Build history of the part. All positions in model axes, mm. A direction names the side the tool comes from. Round coordinates to 2 decimals unless told otherwise and drop trailing zeros. Order: outer loops, then holes, each group sorted by start corner. A loop starts at its lowest first (then second) coordinate and runs counter-clockwise, first axis right, second up. Notation, with made-up numbers: (-22, 85.5) -> (-4, 85.5) arc R31 ccw to (-4, 112.5) -> close; hole circle Ø8 at (89, 73). An arc over 180 degrees is marked (long way). Answer as a JSON object with one key per item and string values.
from build123d import *

# Parameters (mm, degrees)
SKETCH1_R           = 38.1
BOSS_EXTRUDE1_DEPTH = 1.1811
SKETCH2_R           = 36.5125
BOSS_EXTRUDE2_DEPTH = 1.1811
SKETCH3_R           = 3.175
CUT_EXTRUDE1_DEPTH  = 54.933292027


with BuildPart() as part:
    # Sketch1 → Boss-Extrude1 (new body)
    with BuildSketch(Plane.YZ):
        with Locations(Location((0, 0, 0), (0, 0, 270))):
            Circle(SKETCH1_R)
    extrude(amount=BOSS_EXTRUDE1_DEPTH)

    # Sketch2 → Boss-Extrude2 (add)
    with BuildSketch(Plane.YZ.offset(1.1811)):
        with Locations(Location((0, 0, 0), (0, 0, 270))):
            Circle(SKETCH2_R)
    extrude(amount=BOSS_EXTRUDE2_DEPTH)

    # Sketch3 → Cut-Extrude1 (cut, through all)
    with BuildSketch(Plane(origin=(0, 0, 0), x_dir=(0, -1, 0), z_dir=(-1, 0, 0))):
        with Locations(Location((0, 0, 0), (0, 0, 90))):
            Circle(SKETCH3_R)
        with Locations(Location((19.05, 0, 0), (0, 0, 90))):
            Circle(SKETCH3_R)
        with Locations(Location((-19.05, 0, 0), (0, 0, 90))):
            Circle(SKETCH3_R)
    extrude(amount=-CUT_EXTRUDE1_DEPTH, mode=Mode.SUBTRACT)


solid = part.part
1) Probe L1, parallel to Y at x = 0.8, z = 0 (3 decimals); L2, parallel to Y at x = 1.7, z = 0 (1 decimal); L3, parallel to Z at x = 1.5, y = 18. List the from-to ranges inside material, lowest first. Write a range as from..to.
Checked values:
{"L1": "y = -38.1..-22.225, -15.875..-3.175, 3.175..15.875, 22.225..38.1", "L2": "y = -36.5..-22.2, -15.9..-3.2, 3.2..15.9, 22.2..36.5", "L3": "z = -31.77..-3, 3..31.77"}
2) Cut at D-D, the plane y = -27. Give the cut face in (x, z), plus the area to 3 significant figures.
Checked values:
{"outline": "(0, -26.88) -> (1.18, -26.88) -> (1.18, -24.58) -> (2.36, -24.58) -> (2.36, 24.58) -> (1.18, 24.58) -> (1.18, 26.88) -> (0, 26.88) -> close", "area": "122 mm²"}
3) Cut at C-C, the plane z = -10. Give the cut face in (x, y), plus the area to 3 significant figures.
Checked values:
{"outline": "(0, -36.76) -> (1.18, -36.76) -> (1.18, -35.12) -> (2.36, -35.12) -> (2.36, 35.12) -> (1.18, 35.12) -> (1.18, 36.76) -> (0, 36.76) -> close", "area": "170 mm²"}
4) Flat gauge pins, fed straight in: pin 1 Ø8 at (y, z) = (-29.5, -26.5) entering from -X; pin 2 Ø5 at (y, z) = (0, 0) entering from -X. Where does each tip first touch, or does it go through?
Checked values:
{"pin 1": "stops at x = 0", "pin 2": "passes through"}
5) Cut at A-A, the plane y = 0. Give the cut face in (x, z) (1 decimal), plus the area to 3 significant figures.
Checked values:
{"outline": "(0, -38.1) -> (1.2, -38.1) -> (1.2, -36.5) -> (2.4, -36.5) -> (2.4, -3.2) -> (0, -3.2) -> close; (0, 3.2) -> (2.4, 3.2) -> (2.4, 36.5) -> (1.2, 36.5) -> (1.2, 38.1) -> (0, 38.1) -> close", "area": "161 mm²"}
6) Which spindle directions (+Z, -Z, +X, -X, +Y, -Y) get a long thin tool onto all of the face, cutting with end or side? Do faces 5 (the face through (1.763, 10.967, -34.826)), 6 (the face through (2.362, -8, 1)). Say none if no direction does.
Checked values:
{"face 5": "+X", "face 6": "+Z, -Z, +X, +Y, -Y"}
7) Cut at B-B, the plane z = 0. Give the cut face in (x, y) (1 decimal), plus the area to 3 significant figures.
Checked values:
{"outline": "(0, -38.1) -> (1.2, -38.1) -> (1.2, -36.5) -> (2.4, -36.5) -> (2.4, -22.2) -> (0, -22.2) -> close; (0, -15.9) -> (2.4, -15.9) -> (2.4, -3.2) -> (0, -3.2) -> close; (0, 3.2) -> (2.4, 3.2) -> (2.4, 15.9) -> (0, 15.9) -> close; (0, 22.2) -> (2.4, 22.2) -> (2.4, 36.5) -> (1.2, 36.5) -> (1.2, 38.1) -> (0, 38.1) -> close", "area": "131 mm²"}
8) Pull direction Y, two halves, no side cores. Call faces 1 (the face through (0.582, -23.183, 30.235)), 2 (the face through (1.16, 15.95, -0.69)), 3 (the face through (0, 1, -8)), 4 (the face through (1.16, -18.1, 3.03)): pulls with the +Y half, pulls with the -Y half, needs draft (parallel to the pull), parting line crosses it, or undercut.
Checked values:
{"face 1": "parting line crosses it", "face 2": "undercut", "face 3": "needs draft", "face 4": "undercut"}
